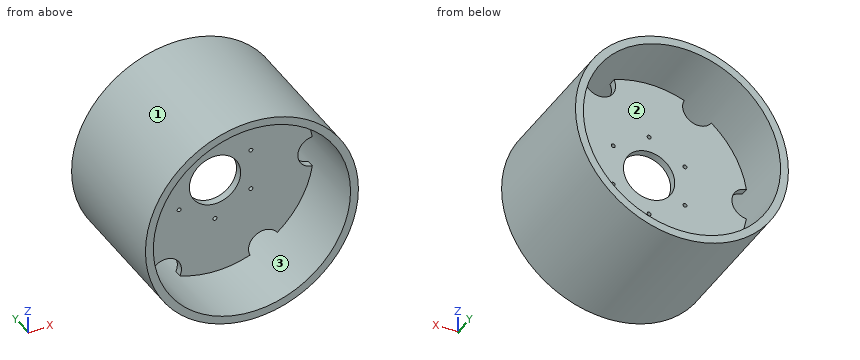
```python
from build123d import *

# Parameters (mm, degrees)
F0_R     = 250
F0_R_2   = 5
F0_R_3   = 65
F1_DEPTH = 10
F3_DEPTH = 20.001
F4_R     = 270
F4_R_2   = 250
F5_DEPTH = 180


with BuildPart() as f1:
    # F0 (on Front) → F1 (new body, symmetric)
    with BuildSketch(Plane.XZ):
        Circle(F0_R)
        with Locations((-90.932667, -52.5)):
            Circle(F0_R_2, mode=Mode.SUBTRACT)
        with Locations((0, -105)):
            Circle(F0_R_2, mode=Mode.SUBTRACT)
        with Locations((90.932667, -52.5)):
            Circle(F0_R_2, mode=Mode.SUBTRACT)
        with Locations((-90.932667, 52.5)):
            Circle(F0_R_2, mode=Mode.SUBTRACT)
        Circle(F0_R_3, mode=Mode.SUBTRACT)
        with Locations((90.932667, 52.5)):
            Circle(F0_R_2, mode=Mode.SUBTRACT)
        with Locations((0, 105)):
            Circle(F0_R_2, mode=Mode.SUBTRACT)
    extrude(amount=F1_DEPTH, both=True)

    # F2 (on face) → F3 (cut, through all)
    with BuildSketch(Plane.XZ.offset(10)):
        with BuildLine():
            ThreePointArc((157.929987, 193.799172), (125, 216.506351), (88.870013, 233.670967))
            ThreePointArc((88.870013, 233.670967), (105, 181.865335), (157.929987, 193.799172))
        make_face()
        with BuildLine():
            ThreePointArc((250, 0), (249.198716, 20), (246.8, 39.871795))
            ThreePointArc((246.8, 39.871795), (210, 0), (246.8, -39.871795))
            ThreePointArc((246.8, -39.871795), (249.198716, -20), (250, 0))
        make_face()
        with BuildLine():
            ThreePointArc((88.870013, -233.670967), (125, -216.506351), (157.929987, -193.799172))
            ThreePointArc((157.929987, -193.799172), (105, -181.865335), (88.870013, -233.670967))
        make_face()
        with BuildLine():
            ThreePointArc((-88.870013, -233.670967), (-105, -181.865335), (-157.929987, -193.799172))
            ThreePointArc((-157.929987, -193.799172), (-125, -216.506351), (-88.870013, -233.670967))
        make_face()
        with BuildLine():
            ThreePointArc((-246.8, -39.871795), (-210, 0), (-246.8, 39.871795))
            ThreePointArc((-246.8, 39.871795), (-250, 0), (-246.8, -39.871795))
        make_face()
        with BuildLine():
            ThreePointArc((-157.929987, 193.799172), (-105, 181.865335), (-88.870013, 233.670967))
            ThreePointArc((-88.870013, 233.670967), (-125, 216.506351), (-157.929987, 193.799172))
        make_face()
    extrude(amount=-F3_DEPTH, mode=Mode.SUBTRACT)

    # F4 (on face) → F5 (join, symmetric)
    with BuildSketch(Plane.XZ.offset(10)):
        Circle(F4_R)
        Circle(F4_R_2, mode=Mode.SUBTRACT)
    extrude(amount=F5_DEPTH, both=True)


solid = f1.part
```
The listing builds one solid part. Answer for the finished solid, in the listing's coordinates (mm). Face numbers are marked on the shaded views. Round coordinates to 2 decimals unless told otherwise and drop trailing zeros. Loops run counter-clockwise (first coordinate to the right, second up) from the corner with the lowest first, then second, coordinate; pieces in that order, holes last.
Q1. Section B-B, the plane x = -120 is taken. Determine the outline of the cut face in (y, z), then the cut area to 3 significant figures.
Q2. Section A-A, the plane z = 0 is taken. Determine the outline of the cut face in (x, y), then the cut area to 3 significant figures.
Q3. For a pull along Z with two mould halves and no side action, classify the marked faces 1, 2 and 3 as released by +Z, released by -Z, zero draft, split by the parting line, or undercut.
Q4. Section C-C, the plane y = 78.5 is taken. Determine the outline of the cut face in (x, z), then the cut area to 3 significant figures.
Q5. Given pin 1 Ø1.5 at (y, z) = (77, -214.5) entering from -X; pin 2 Ø13 at (x, z) = (90.93, -52.5) entering from +Y; pin 3 Ø2 at (x, y) = (150.5, -93) entering from +Z, each flat-ended and moving along its own axis, determine where each tip first touches the part or whether it passes through.
Q6. Section D-D, the plane x = 109 is taken. Determine the outline of the cut face in (y, z).
Q7. Find the intervals of material crossed by line 1 (Z direction, x = 0, y = 0); line 2 (X direction, y = 6.5, z = -217); line 3 (Z direction, x = 0, y = -80), in increasing order.
Completed:
1. outline: (-190, -241.87) - (170, -241.87) - (170, -219.32) - (-190, -219.32) - close; (-190, 219.32) - (170, 219.32) - (170, 241.87) - (-190, 241.87) - close; (-10, -176.82) - (10, -176.82) - (10, 176.82) - (-10, 176.82) - close
1. area: 23,300 mm2
2. outline: (-270, -190) - (-250, -190) - (-250, 170) - (-270, 170) - close; (-210, -10) - (-65, -10) - (-65, 10) - (-210, 10) - close; (65, -10) - (210, -10) - (210, 10) - (65, 10) - close; (250, -190) - (270, -190) - (270, 170) - (250, 170) - close
2. area: 20,200 mm2
3. face 1: split by the parting line
3. face 2: undercut
3. face 3: undercut
4. outline: circle Ø540 at (0, 0); hole circle Ø500 at (0, 0)
4. area: 32,700 mm2
5. pin 1: stops at x = -164.96
5. pin 2: stops at y = 10
5. pin 3: stops at z = 224.83
6. outline: (-190, -247.02) - (170, -247.02) - (170, -224.99) - (-190, -224.99) - close; (-190, 224.99) - (170, 224.99) - (170, 247.02) - (-190, 247.02) - close; (-10, -179.85) - (10, -179.85) - (10, 179.85) - (-10, 179.85) - close
7. line 1: z = -270 to -110, -100 to -65, 65 to 100, 110 to 270
7. line 2: x = -160.66 to -124.14, -85 to 85, 124.14 to 160.66
7. line 3: z = -270 to -250, 250 to 270
